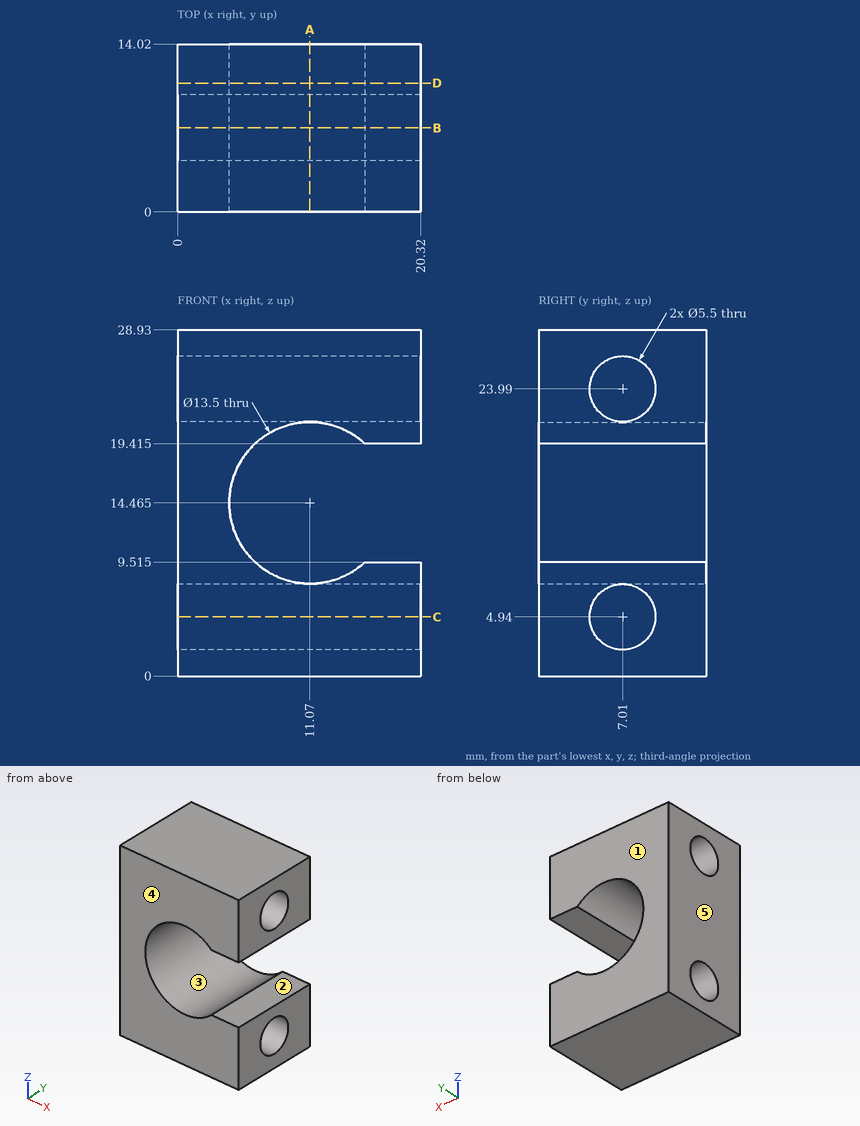
Study the drawing (mm; zero at the part's minimum x, y, z) and answer. A direction names the side the tool comes from. Coordinates: 2 decimals unless noted, no trailing zeros. Loops run counter-clockwise (first coordinate to the right, second up) from the corner with the lowest first, then second, coordinate; pieces in that order, holes last. Notation, with made-up numbers: (-29.75, 70) -> (-8.75, 70) arc R28 ccw to (-8.75, 95) -> close; hole circle Ø11 at (73.5, 26). An arc over 180 degrees is marked (long way). Answer in a Markdown table with one row per item. Add a question column.
1. The part is cut by section A-A, the plane x = 11.07. Write down the section's boundary in (y, z) (3 decimals).
2. For the marked faces 1 and 2, determine the directions among +Z, -Z, +X, -X, +Y, -Y from which every point of the face is accessible in a straight line to the end or side of a thin tool.
3. Consider line 1 (Z direction, x = 11.07, y = 10.5) (3 decimals); line 2 (Z direction, x = 11.25, y = 6); line 3 (Z direction, x = 11.07, y = 5) (3 decimals). Determine where each line is inside the solid, lowest interval first. Write a range as [from, to].
4. Determine the mould class of the marked faces 3, 4 and 5 for opening direction X: +X half, -X half, draft (parallel to the pull), parting line (faces both ways), or undercut.
5. Flat-ended cylindrical pins translate along their axes: P1, Ø1, axis at y = 5, z = 17, coming from the +X side; P2, Ø7, axis at y = 7.01, z = 23.99, coming from the -X side. Find the tip coordinate at first contact, or state that the pin passes through.
6. The part is cut by section D-D, the plane y = 10.75. Write down the section's boundary in (x, z) (3 decimals), then the cut area to 3 significant figures.
7. The part is cut by section B-B, the plane y = 7.01. Write down the section's boundary in (x, z) (3 decimals).
8. The part is cut by section C-C, the plane z = 4.94. Write down the section's boundary in (x, y), then the cut area to 3 significant figures.
Answer below:
| question | item | result |
|---|---|---|
| 1 | outline | (0, 0) -> (14.02, 0) -> (14.02, 7.715) -> (0, 7.715) -> close; (0, 21.215) -> (14.02, 21.215) -> (14.02, 28.93) -> (0, 28.93) -> close; hole circle Ø5.5 at (7.01, 4.94); hole circle Ø5.5 at (7.01, 23.99) |
| 2 | face 1 | +Z, -Z, +X, -X, +Y |
| 2 | face 2 | +X, +Y, -Y |
| 3 | line 1 | [0, 7.715], [21.215, 28.93] |
| 3 | line 2 | [0, 2.38], [7.5, 7.72], [21.21, 21.43], [26.55, 28.93] |
| 3 | line 3 | [0, 3.063], [6.817, 7.715], [21.215, 22.113], [25.867, 28.93] |
| 4 | face 3 | undercut |
| 4 | face 4 | draft |
| 4 | face 5 | -X half |
| 5 | P1 | x = 5.04 |
| 5 | P2 | x = 0 |
| 6 | outline | (0, 0) -> (20.32, 0) -> (20.32, 9.515) -> (15.659, 9.515) arc R6.75 cw (long way) to (15.659, 19.415) -> (20.32, 19.415) -> (20.32, 28.93) -> (0, 28.93) -> close |
| 6 | area | 413 mm2 |
| 7 | outline | (0, 0) -> (20.32, 0) -> (20.32, 2.19) -> (0, 2.19) -> close; (0, 7.69) -> (20.32, 7.69) -> (20.32, 9.515) -> (15.659, 9.515) arc R6.75 cw (long way) to (15.659, 19.415) -> (20.32, 19.415) -> (20.32, 21.24) -> (0, 21.24) -> close; (0, 26.74) -> (20.32, 26.74) -> (20.32, 28.93) -> (0, 28.93) -> close |
| 8 | outline | (0, 0) -> (20.32, 0) -> (20.32, 4.26) -> (0, 4.26) -> close; (0, 9.76) -> (20.32, 9.76) -> (20.32, 14.02) -> (0, 14.02) -> close |
| 8 | area | 173 mm2 |
